Build history of the part. All positions in model axes, mm. Face numbers are marked on the shaded views. A direction names the side the tool comes from. Round coordinates to 2 decimals unless told otherwise and drop trailing zeros. Write each loop counter-clockwise with the first axis right and the second up, starting at its lowest first coordinate (ties: lowest second). Pieces come first, ordered by that corner, then holes. Notation, with made-up numbers: M 35.25,88.5 L 68.25,88.5 A27 ccw 68.25,105.5 Z; hole C 67.5,32 d6. An arc over 180 degrees is marked long. Use a Markdown table: item, result.
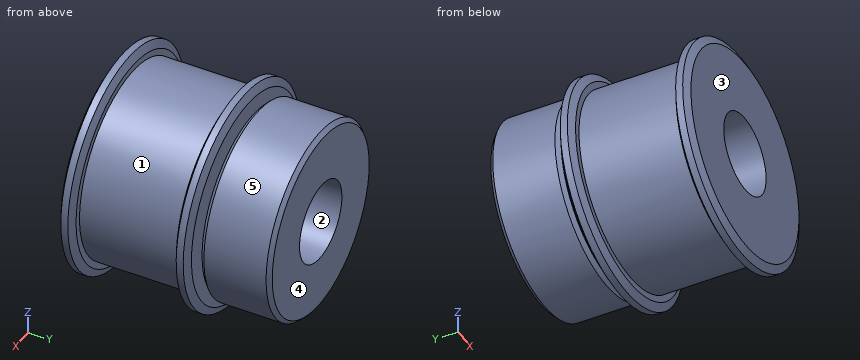
from build123d import *

# Parameters (mm, degrees)
F2_C1_SIZE2 = 0.4
F2_C1_SIZE  = 0.8
F2_C2_SIZE2 = 0.8
F2_C2_SIZE  = 0.4
F2_C3_SIZE2 = 0.8
F2_C3_SIZE  = 0.4
F3_SIZE2    = 0.4
F3_SIZE     = 0.8
F4_SIZE     = 0.4


with BuildPart() as f1:
    # F0 (on Right) → F1 (revolve)
    with BuildSketch(Plane.YZ):
        Polygon((-10.25, 11), (-10.25, 4), (10.25, 4), (10.25, 9.55), (3.25, 9.55), (3.25, 6.35), (2.75, 6.35), (2.75, 11), (1.25, 11), (1.25, 9.55), (-8.75, 9.55), (-8.75, 11), align=None)
    revolve(axis=Axis((0, -3.1587743408, 0), (0, -1, 0)))

    # F2: chamfer of 0.4 x 0.8 on 3 edges, made by hand

    # F2_c1
    f2_c1_edges = [f1.edges().sort_by_distance(p)[0] for p in [
        (0, -10.25, -11),
    ]]
    f2_c1_side = f1.faces().sort_by_distance((0, -10.25, -10.992))[0]
    chamfer(f2_c1_edges, length=F2_C1_SIZE, length2=F2_C1_SIZE2, reference=f2_c1_side)

    # F2_c2
    f2_c2_edges = [f1.edges().sort_by_distance(p)[0] for p in [
        (0, 2.75, -11),
    ]]
    f2_c2_side = f1.faces().sort_by_distance((0, 2.742, -11))[0]
    chamfer(f2_c2_edges, length=F2_C2_SIZE, length2=F2_C2_SIZE2, reference=f2_c2_side)

    # F2_c3
    f2_c3_edges = [f1.edges().sort_by_distance(p)[0] for p in [
        (0, 1.25, -11),
    ]]
    f2_c3_side = f1.faces().sort_by_distance((0, 1.258, -11))[0]
    chamfer(f2_c3_edges, length=F2_C3_SIZE, length2=F2_C3_SIZE2, reference=f2_c3_side)

    # F3
    f3_edges = [f1.edges().sort_by_distance(p)[0] for p in [
        (0, -8.75, -11),
    ]]
    chamfer(f3_edges, length=F3_SIZE, length2=F3_SIZE2)

    # F4
    f4_edges = [f1.edges().sort_by_distance(p)[0] for p in [
        (0, 3.25, -9.55),
        (0, 10.25, -9.55),
    ]]
    chamfer(f4_edges, length=F4_SIZE)


solid = f1.part
Q1. Drill centre lines: L1, parallel to Y at x = -10, z = -0.5; L2, parallel to Z at x = 0, y = 5.25. Where is each one in solid material? Low to high.
Response values:
| item | result |
|---|---|
| L1 | y = -10.25 to -8.75, 1.25 to 2.75 |
| L2 | z = -9.55 to -4, 4 to 9.55 |
Q2. Which spindle directions (+Z, -Z, +X, -X, +Y, -Y) get a long thin tool onto all of the face, cutting with end or side? Do the marked faces 4 and 5. Say none if no direction does.
Response values:
| item | result |
|---|---|
| face 4 | +Z, -Z, +X, -X, +Y |
| face 5 | +Y |
Q3. Drop flat-ended pins along their axis: P1, Ø3, axis at x = 8, y = -6, coming from the -Z side; P2, Ø3, axis at y = 6.5, z = -2, coming from the -X side; P3, Ø6, axis at x = -7, y = 4, coming from the +Z side; P4, Ø6.5, axis at x = 0, z = 0, coming from the -Y side. Give the stop position or say it passes through.
Response values:
| item | result |
|---|---|
| P1 | stops at z = -7 |
| P2 | stops at x = -9.54 |
| P3 | stops at z = 10.04 |
| P4 | passes through |
Q4. Two-plate mould, pull along Y, no slides. Class the marked faces 1, 2 and 3: +Y half, -Y half, draft (parallel to the pull), parting line (faces both ways), or undercut.
Response values:
| item | result |
|---|---|
| face 1 | undercut |
| face 2 | draft |
| face 3 | -Y half |
Q5. Cut at A-A on y = -6. Give the cut face in (x, z).
Response values:
| item | result |
|---|---|
| outline | C 0,0 d19.1; hole C 0,0 d8 |
